from build123d import *

# Parameters (mm, degrees)
SKETCH1_R                                       = 17.5
BOSS_EXTRUDE9_DEPTH                             = 25.5
BOSS_EXTRUDE10_DEPTH                            = 15.4
BOSS_EXTRUDE10_DEPTH_BACK                       = 25.5
CSK_FOR_M3_FLAT_HEAD_MACHINE_SCREW1_D           = 3.6
CSK_FOR_M3_FLAT_HEAD_MACHINE_SCREW1_CSINK_D     = 6.3
CSK_FOR_M3_FLAT_HEAD_MACHINE_SCREW1_CSINK_ANGLE = 90
CSK_FOR_M3_FLAT_HEAD_MACHINE_SCREW2_D           = 3.6
CSK_FOR_M3_FLAT_HEAD_MACHINE_SCREW2_CSINK_D     = 6.3
CSK_FOR_M3_FLAT_HEAD_MACHINE_SCREW2_CSINK_ANGLE = 90
BOSS_EXTRUDE11_DEPTH                            = 15.4
CUT_EXTRUDE3_REACH                              = 549.129
SKETCH17_R                                      = 1.8


with BuildPart() as part:
    # Sketch1 → Boss-Extrude9 (new body)
    with BuildSketch(Plane.XY):
        with BuildLine():
            ThreePointArc((-19.6, 18.153395679), (0, 37.753395679), (19.6, 18.153395679))
            ThreePointArc((19.6, 18.153395679), (0, -1.446604321), (-19.6, 18.153395679))
        make_face()
        with Locations((0, 18.153395679)):
            Circle(SKETCH1_R, mode=Mode.SUBTRACT)
    extrude(amount=-BOSS_EXTRUDE9_DEPTH)

    # Sketch1<15> → Boss-Extrude10 (add, two sides: drawn at the far end of the back side and taken through both)
    with BuildSketch(Plane.XY.offset(-BOSS_EXTRUDE10_DEPTH_BACK)):
        with BuildLine():
            Line((-23, -1.846604321), (-38, -1.846604321))
            Line((-38, -1.846604321), (-38, -6.846604321))
            Line((-38, -6.846604321), (38, -6.846604321))
            Line((38, -6.846604321), (38, -1.846604321))
            Line((38, -1.846604321), (23, -1.846604321))
            Line((23, -1.846604321), (19.6, 18.153395679))
            ThreePointArc((19.6, 18.153395679), (0, -1.446604321), (-19.6, 18.153395679))
            Line((-19.6, 18.153395679), (-23, -1.846604321))
        make_face()
    extrude(amount=BOSS_EXTRUDE10_DEPTH + BOSS_EXTRUDE10_DEPTH_BACK)

    # CSK for M3 Flat Head Machine Screw1 (through all)
    with Locations(Plane(origin=(0, -1.846604321, 0), x_dir=(1, 0, 0), z_dir=(0, 1, 0))):
        with Locations((-30.5, 15.5), (-30.5, -5.4)):
            CounterSinkHole(CSK_FOR_M3_FLAT_HEAD_MACHINE_SCREW1_D / 2, CSK_FOR_M3_FLAT_HEAD_MACHINE_SCREW1_CSINK_D / 2, counter_sink_angle=CSK_FOR_M3_FLAT_HEAD_MACHINE_SCREW1_CSINK_ANGLE)

    # CSK for M3 Flat Head Machine Screw2 (through all)
    with Locations(Plane(origin=(0, -1.846604321, 0), x_dir=(1, 0, 0), z_dir=(0, 1, 0))):
        with Locations((30.5, -5.4), (30.5, 15.5)):
            CounterSinkHole(CSK_FOR_M3_FLAT_HEAD_MACHINE_SCREW2_D / 2, CSK_FOR_M3_FLAT_HEAD_MACHINE_SCREW2_CSINK_D / 2, counter_sink_angle=CSK_FOR_M3_FLAT_HEAD_MACHINE_SCREW2_CSINK_ANGLE)

    # Sketch1<19> → Boss-Extrude11 (add)
    with BuildSketch(Plane.XY):
        with BuildLine():
            ThreePointArc((-19.6, 18.153395679), (0, -1.446604321), (19.6, 18.153395679))
            Line((19.6, 18.153395679), (17, 18.153395679))
            ThreePointArc((17, 18.153395679), (0, 1.153395679), (-17, 18.153395679))
            Line((-17, 18.153395679), (-19.6, 18.153395679))
        make_face()
    extrude(amount=BOSS_EXTRUDE11_DEPTH)

    # Sketch17 → Cut-Extrude3 (cut, up to next)
    with BuildSketch(Plane(origin=(-499.24894984, 9.974554812, -84.308871479), x_dir=(0.050830850863694654, -0.0009181581696580717, 0.9987068546806156), z_dir=(0.0360908865319125, 0.9993480899541042, -0.0009181581696581681)), mode=Mode.PRIVATE) as cut_extrude3_sk1:
        with Locations((92.5, 462.5)):
            Circle(SKETCH17_R)
    cut_extrude3_tool1 = extrude(cut_extrude3_sk1.sketch, amount=-CUT_EXTRUDE3_REACH, mode=Mode.PRIVATE) & part.part
    # Sketch17 → Cut-Extrude3 (cut, up to next)
    with BuildSketch(Plane(origin=(-499.24894984, 9.974554812, -84.308871479), x_dir=(0.050830850863694654, -0.0009181581696580717, 0.9987068546806156), z_dir=(0.0360908865319125, 0.9993480899541042, -0.0009181581696581681)), mode=Mode.PRIVATE) as cut_extrude3_sk2:
        with Locations((113.4, 462.5)):
            Circle(SKETCH17_R)
    cut_extrude3_tool2 = extrude(cut_extrude3_sk2.sketch, amount=-CUT_EXTRUDE3_REACH, mode=Mode.PRIVATE) & part.part
    add(cut_extrude3_tool1.solids().sort_by_distance((-32.946684, -6.80241, -15.437756))[0], mode=Mode.SUBTRACT)
    add(cut_extrude3_tool2.solids().sort_by_distance((-31.884319, -6.821599, 5.435217))[0], mode=Mode.SUBTRACT)


solid = part.part
Source: CAD feature listing. Evaluate the final solid. Frame: model axes, mm. A direction names the side the tool comes from. Round coordinates to 2 decimals unless told otherwise and drop trailing zeros. Write each loop counter-clockwise with the first axis right and the second up, starting at its lowest first coordinate (ties: lowest second). Pieces come first, ordered by that corner, then holes. Notation, with made-up numbers: M 13.5,59.5 L 26.5,59.5 A27 cw 26.5,75.5 Z; hole C 47.25,70.25 d5. An arc over 180 degrees is marked long. One line per item, written item: value. Start each with the question number.
Item 1: Set-up query: faces 1 (the cylindrical face through (-3.79, 1.07, -12.57)), 2 (the flat face through (-30, -1.847, -5)), 3 (the flat face through (0, 36, 0)), 4 (the flat face through (-1, -6.847, -5)), 5 (the flat face through (-3, 0.7, -25.5)). Return all of +Z, -Z, +X, -X, +Y, -Y with unobstructed straight access to the full face (end or side cutting, diameter ignored); none if empty.
Item 2: Section query C-C (z = 13). Return the cut outline in (x, y).
Item 3: Section query B-B (y = 31). Return the cut outline in (x, z).
Item 4: Ray query, L1, parallel to X at y = -5.1, z = 5.4; L2, parallel to Z at x = -30.5, y = -6.1; L3, parallel to X at y = 18.5, z = -9. Return the intervals inside material, ascending. Write a range as from..to.
Item 5: Mould query, pull axis X, two halves, no side actions, for faces 6 (the flat face through (18, 18.153, 8)), 7 (the flat face through (38, -4, -5)), 8 (the cylindrical face through (28.837, -5.047, 6.089)). Classes: pulls with the +X half, pulls with the -X half, needs draft (parallel to the pull), parting line crosses it, or undercut.
Item 6: Pin query (flat end, axial travel): pin 1 (4 mm diameter, centred on x = -30.5, z = -15.5, fed in from +Y); pin 2 (9 mm diameter, centred on x = 2, y = 6.5, fed in from -Z); pin 3 (5 mm diameter, centred on x = 12, y = 27.5, fed in from +Z); pin 4 (1.3 mm diameter, centred on x = 19, z = 10, fed in from +Y). Return the tip coordinate at first contact, or that it passes through.
Item 7: Section query A-A (x = 0). Return the cut outline in (y, z).
Item 8: Section query D-D (z = -8). Return the cut outline in (x, y), plus the area to 3 significant figures.
Result set:
1. face 1: -Z
1. face 2: +Z, -Z, -X, +Y
1. face 3: +Z, +X, -X, +Y
1. face 4: +Z, -Z, +X, -X, -Y
1. face 5: -Z, +X, -X, +Y, -Y
2. outline: M -38,-6.85 L 38,-6.85 L 38,-1.85 L 23,-1.85 L 19.6,18.15 L 17,18.15 A17 cw -17,18.15 L -19.6,18.15 L -23,-1.85 L -38,-1.85 Z
3. outline: M -14.8,-25.5 L -11.88,-25.5 L -11.88,0 L -14.8,0 Z; M 11.88,-25.5 L 14.8,-25.5 L 14.8,0 L 11.88,0 Z
4. L1: x = -38..-32.3, -28.7..28.7, 32.3..38
4. L2: z = -25.5..-17.3, -13.7..3.6, 7.2..15.4
4. L3: x = -19.6..-17.5, 17.5..19.6
5. face 6: needs draft
5. face 7: pulls with the +X half
5. face 8: undercut
6. pin 1: stops at y = -3
6. pin 2: passes through
6. pin 3: stops at z = 0
6. pin 4: stops at y = 18.15
7. outline: M -6.85,-25.5 L 0.65,-25.5 L 0.65,0 L 1.15,0 L 1.15,15.4 L -6.85,15.4 Z; M 35.65,-25.5 L 37.75,-25.5 L 37.75,0 L 35.65,0 Z
8. outline: M -38,-6.85 L 38,-6.85 L 38,-1.85 L 23,-1.85 L 19.6,18.15 A19.6 ccw -19.6,18.15 L -23,-1.85 L -38,-1.85 Z; hole C 0,18.15 d35
8. area: 873 mm²
